```python
from build123d import *

# Parameters (mm, degrees)
ESQUISSE1_W        = 59.8
ESQUISSE1_H        = 59.8
BOSS_EXTRU_1_DEPTH = 5
ESQUISSE2_W        = 45.3
ESQUISSE2_H        = 45.3
BOSS_EXTRU_2_DEPTH = 24.3
CONG_1_R           = 3.7
ESQUISSE6_W        = 56.2
ESQUISSE6_H        = 56.2
BOSS_EXTRU_4_DEPTH = 10
BOSS_EXTRU_4_TAPER = 45


with BuildPart() as part:
    # Esquisse1 → Boss.-Extru.1 (new body)
    with BuildSketch(Plane.XY):
        Rectangle(ESQUISSE1_W, ESQUISSE1_H)
    extrude(amount=BOSS_EXTRU_1_DEPTH)

    # Esquisse2 → Boss.-Extru.2 (add)
    with BuildSketch(Plane.XY):
        Rectangle(ESQUISSE2_W, ESQUISSE2_H)
    extrude(amount=BOSS_EXTRU_2_DEPTH)

    # Congé1
    cong_1_edges = [part.edges().sort_by_distance(p)[0] for p in [
        (29.9, -29.9, 2.5),
        (-29.9, -29.9, 2.5),
        (-29.9, 29.9, 2.5),
        (29.9, 29.9, 2.5),
    ]]
    fillet(cong_1_edges, radius=CONG_1_R)

    # Esquisse6 → Boss.-Extru.4 (add)
    with BuildSketch(Plane.XY.offset(10)):
        Rectangle(ESQUISSE6_W, ESQUISSE6_H)
    extrude(amount=BOSS_EXTRU_4_DEPTH, taper=BOSS_EXTRU_4_TAPER)


solid = part.part
```
Can you work these out from the model? Positions are in its coordinate system, mm. A direction names the side the tool comes from. Give positions to 0.01 mm unless a question says otherwise; leave off trailing zeros. Loops run counter-clockwise (first coordinate to the right, second up) from the corner with the lowest first, then second, coordinate; pieces in that order, holes last. Notation, with made-up numbers: M 30.25,-5 L 70.25,-5 A29 cw 70.25,25 Z; hole C -24.5,38.5 d3. An arc over 180 degrees is marked long. Use one line per item in the form item = value. Start each with the question number.
(1) Thinking about a two-plate mould opening in Z: for faces 1 (the flat face through (0, 22.65, 7)), 2 (the flat face through (-0.4, 25.4, 12.7)), 3 (the flat face through (0, -22.65, 20)), which applies, released by +Z, released by -Z, zero draft, split by the parting line, or undercut?
(2) I'm going to push flat-ended pins straight in: P1, Ø5, axis at y = -16.5, z = 10, coming from the -X side; P2, Ø2.5, axis at x = 6.5, z = 8.5, coming from the +Y side; P3, Ø2.5, axis at x = 11, z = 7, coming from the -Y side. Where does each tip first touch, or does it pass through?
(3) On a 3-axis mill with a long thin cutter (end or side, diameter ignored), from which of +Z, -Z, +X, -X, +Y, -Y can I reach the whole of each face in a straight line? I mean faces 4 (the flat face through (-22.65, 0, 20)), 5 (the flat face through (22.65, 0, 20)), 6 (the flat face through (-22.65, 0, 7)). Say none if no direction works.
(4) I want a section at D-D, the plane z = 8.25. Write out the boundary of the cut face in (x, y), and give its area (3 significant figures).
(5) Please list where these lines run through material, in increasing order: line 1 (X direction, y = 22, z = 9.75); line 2 (Z direction, x = -24, y = -9.5).
(6) I want a section at C-C, the plane z = 13.75. Write out the boundary of the cut face in (x, y).
(7) I want a section at A-A, the plane x = 11.5. Write out the boundary of the cut face in (y, z), and give its area (3 significant figures).
Worked out:
q1.face_1 = undercut
q1.face_2 = released by +Z
q1.face_3 = zero draft
q2.P1 = -28.1
q2.P2 = 22.65
q2.P3 = -22.65
q3.face_4 = +Z, -X, +Y, -Y
q3.face_5 = +Z, +X, +Y, -Y
q3.face_6 = -X, +Y, -Y
q4.outline = M -22.65,-22.65 L 22.65,-22.65 L 22.65,22.65 L -22.65,22.65 Z
q4.area = 2,050 mm²
q5.line_1 = -22.65 to 22.65
q5.line_2 = 0 to 5, 10 to 14.1
q6.outline = M -24.35,-24.35 L 24.35,-24.35 L 24.35,24.35 L -24.35,24.35 Z
q7.outline = M -29.9,0 L 29.9,0 L 29.9,5 L 22.65,5 L 22.65,10 L 28.1,10 L 22.65,15.45 L 22.65,24.3 L -22.65,24.3 L -22.65,15.45 L -28.1,10 L -22.65,10 L -22.65,5 L -29.9,5 Z
q7.area = 1,200 mm²
